```python
from build123d import *

# Parameters (mm, degrees)
F0_W      = 30
F0_H      = 30
F1_DEPTH  = 15
F2_SIZE   = 9.5
F3_R      = 3
F4_DEPTH  = 2.5
F5_R      = 3
F6_DEPTH  = 2.5
F7_R      = 3
F8_DEPTH  = 2.5
F9_R      = 3
F10_DEPTH = 2.5
F11_R     = 3
F12_DEPTH = 2.5
F13_R     = 3
F14_DEPTH = 2.5
F15_R     = 3
F16_DEPTH = 2.5
F17_R     = 3
F18_DEPTH = 2.5


with BuildPart() as f1:
    # F0 (on Front) → F1 (new body, symmetric)
    with BuildSketch(Plane.XZ):
        Rectangle(F0_W, F0_H)
    extrude(amount=F1_DEPTH, both=True)

    # F2
    f2_edges = [f1.edges().sort_by_distance(p)[0] for p in [
        (0, 15, -15),
        (0, 15, 15),
        (15, 15, 0),
        (-15, 15, 0),
        (15, 0, 15),
        (0, -15, 15),
        (-15, 0, 15),
        (-15, -15, 0),
        (15, -15, 0),
        (0, -15, -15),
        (-15, 0, -15),
        (15, 0, -15),
    ]]
    chamfer(f2_edges, length=F2_SIZE)

    # F3 (on face) → F4 (cut)
    with BuildSketch(Plane(origin=(-8.666667, 8.666667, 8.666667), x_dir=(-0.408248, -0.816497, 0.408248), z_dir=(-0.57735, 0.57735, 0.57735))):
        Circle(F3_R)
    extrude(amount=-F4_DEPTH, mode=Mode.SUBTRACT)

    # F5 (on face) → F6 (cut)
    with BuildSketch(Plane(origin=(8.666667, 8.666667, -8.666667), x_dir=(-0.408248, 0.816497, 0.408248), z_dir=(0.57735, 0.57735, -0.57735))):
        Circle(F5_R)
    extrude(amount=-F6_DEPTH, mode=Mode.SUBTRACT)

    # F7 (on face) → F8 (cut)
    with BuildSketch(Plane(origin=(-8.666667, 8.666667, -8.666667), x_dir=(-0.408248, -0.816497, -0.408248), z_dir=(-0.57735, 0.57735, -0.57735))):
        Circle(F7_R)
    extrude(amount=-F8_DEPTH, mode=Mode.SUBTRACT)

    # F9 (on face) → F10 (cut)
    with BuildSketch(Plane(origin=(-8.666667, -8.666667, 8.666667), x_dir=(0.816497, -0.408248, 0.408248), z_dir=(-0.57735, -0.57735, 0.57735))):
        Circle(F9_R)
    extrude(amount=-F10_DEPTH, mode=Mode.SUBTRACT)

    # F11 (on face) → F12 (cut)
    with BuildSketch(Plane(origin=(8.666667, -8.666667, 8.666667), x_dir=(0.816497, 0.408248, -0.408248), z_dir=(0.57735, -0.57735, 0.57735))):
        Circle(F11_R)
    extrude(amount=-F12_DEPTH, mode=Mode.SUBTRACT)

    # F13 (on face) → F14 (cut)
    with BuildSketch(Plane(origin=(-8.666667, -8.666667, -8.666667), x_dir=(0.408248, -0.816497, 0.408248), z_dir=(-0.57735, -0.57735, -0.57735))):
        Circle(F13_R)
    extrude(amount=-F14_DEPTH, mode=Mode.SUBTRACT)

    # F15 (on face) → F16 (cut)
    with BuildSketch(Plane(origin=(8.666667, 8.666667, 8.666667), x_dir=(-0.408248, 0.816497, -0.408248), z_dir=(0.57735, 0.57735, 0.57735))):
        Circle(F15_R)
    extrude(amount=-F16_DEPTH, mode=Mode.SUBTRACT)

    # F17 (on face) → F18 (cut)
    with BuildSketch(Plane(origin=(8.666667, -8.666667, -8.666667), x_dir=(0.408248, 0.816497, -0.408248), z_dir=(0.57735, -0.57735, -0.57735))):
        Circle(F17_R)
    extrude(amount=-F18_DEPTH, mode=Mode.SUBTRACT)


solid = f1.part
```
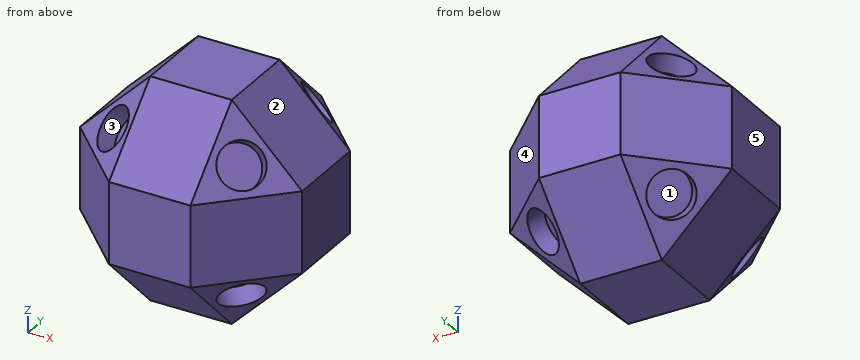
Work out the finished part from the listing and answer in its coordinate system (mm). Face numbers are marked on the shaded views. A direction names the side the tool comes from. Give positions to 0.01 mm unless a question says otherwise; leave off trailing zeros. Loops run counter-clockwise (first coordinate to the right, second up) from the corner with the lowest first, then second, coordinate; pieces in that order, holes last. Notation, with made-up numbers: (-20, 45) -> (-3, 45) arc R25 cw to (-3, 76) -> close; hole circle Ø1 at (61, 44). An arc over 180 degrees is marked (long way). Write item = value, one per line. Start each with the question number.
(1) Given pin 1 Ø3 at (y, z) = (-10.5, 2.5) entering from -X; pin 2 Ø8 at (y, z) = (7.5, -11) entering from +X; pin 3 Ø5 at (x, z) = (-3.5, -10) entering from -Y; pin 4 Ø10 at (y, z) = (-9, -0.5) entering from +X, each flat-ended and moving along its own axis, determine where each tip first touches the part or whether it passes through.
(2) Find section A-A on y = -2. Give the vertices of the cut face in (x, z), and give its area (4 significant figures).
(3) The mould has two halves that part along Y. Classify the marked faces 3, 4 and 5: +Y half, -Y half, draft (parallel to the pull), parting line (faces both ways), or undercut.
(4) Which of the six approach directions +Z, -Z, +X, -X, +Y, -Y give full straight-line access (tool end or side, diameter ignored) to the marked faces 1 and 2?
(5) Find the intervals of material crossed by probe 1 along X at (y, z) = (-8, 6.75); probe 2 along Y at (x, z) = (-9.25, 1.25); probe 3 along Z at (x, y) = (2.5, 12.25), in increasing order. Write a range as from..to.
From the geometry:
q1.pin_1 = -11.5
q1.pin_2 = 12.96
q1.pin_3 = -13
q1.pin_4 = 15
q2.outline = (-15, -5.5) -> (-5.5, -15) -> (5.5, -15) -> (15, -5.5) -> (15, 5.5) -> (5.5, 15) -> (-5.5, 15) -> (-15, 5.5) -> close
q2.area = 719.5 mm^2
q3.face_3 = undercut
q3.face_4 = +Y half
q3.face_5 = draft
q4.face_1 = none
q4.face_2 = +Z, +X, +Y, -Y
q5.probe_1 = -11.25..-10.89, -6.92..6.92, 10.89..11.25
q5.probe_2 = -11.25..11.25
q5.probe_3 = -8.25..8.25
